from build123d import *

# Parameters (mm, degrees)
SKETCH2_R               = 1
CUT_EXTRUDE2_DEPTH      = 8.5
CUT_EXTRUDE2_DEPTH_BACK = 8.5


with BuildPart() as part:
    # Sketch1 → Revolve2 (revolve)
    with BuildSketch(Plane.XY):
        Polygon((-16.067192276, 0), (38.932807724, 0), (38.932807724, 2.992227979), (-12.067192276, 2.992227979), (-12.067192276, 7.5), (-16.067192276, 7.5), align=None)
    revolve(axis=Axis((-16.067192276, 0, 0), (1, 0, 0)))

    # Sketch2 → Cut-Extrude2 (cut, two sides)
    with BuildSketch(Plane.XY) as cut_extrude2_sk:
        with Locations((35.91188951, 0)):
            Circle(SKETCH2_R)
    extrude(amount=CUT_EXTRUDE2_DEPTH, mode=Mode.SUBTRACT)
    extrude(cut_extrude2_sk.sketch, amount=-CUT_EXTRUDE2_DEPTH_BACK, mode=Mode.SUBTRACT)


solid = part.part
Source: CAD feature listing. Evaluate the final solid. Frame: model axes, mm. A direction names the side the tool comes from. Round coordinates to 2 decimals unless told otherwise and drop trailing zeros. Order: outer loops, then holes, each group sorted by start corner. A loop starts at its lowest first (then second) coordinate and runs counter-clockwise, first axis right, second up. Notation, with made-up numbers: (59, -17.5) - (86, -17.5) arc R13 cw to (86, 1.5) - close; hole circle Ø5 at (63.25, 3). An arc over 180 degrees is marked (long way). Use a Markdown table: item, result. Add a question column.
1. Section query B-B (z = -2.5). Return the cut outline in (x, y).
2. Section query D-D (z = 2). Return the cut outline in (x, y).
3. Section query C-C (y = -4.5). Return the cut outline in (x, z), then the cut area to 3 significant figures.
4. Line query: probe 1 along X at (y, z) = (0, -0.75); probe 2 along X at (y, z) = (2.25, -5.25); probe 3 along Z at (x, y) = (-1, 0.25). Output: solid intervals per line, ascending.
5. Set-up query: faces 1 (the cylindrical face through (13.076, 2.854, 0.899)), 2 (the flat face through (-16.067, 0, 0)). Return all of +Z, -Z, +X, -X, +Y, -Y with unobstructed straight access to the full face (end or side cutting, diameter ignored); none if empty.
6. Section query A-A (y = 0). Return the cut outline in (x, z), then the cut area to 3 significant figures.
7. First-contact query: pin 1 (5 mm diameter, centred on x = -2, z = 0, fed in from +Y); pin 2 (4 mm diameter, centred on x = 13, z = -0.5, fed in from -Y); pin 3 (8 mm diameter, centred on y = -2.5, z = 5, fed in from +X); pin 4 (3 mm diameter, centred on x = 35.91, y = 0, fed in from -Z). Flat tips, straight axial feed; report the tip coordinate or a pass-through.
Derived:
| question | item | result |
|---|---|---|
| 1 | outline | (-16.07, -7.07) - (-12.07, -7.07) - (-12.07, -1.64) - (38.93, -1.64) - (38.93, 1.64) - (-12.07, 1.64) - (-12.07, 7.07) - (-16.07, 7.07) - close; hole circle Ø2 at (35.91, 0) |
| 2 | outline | (-16.07, -7.23) - (-12.07, -7.23) - (-12.07, -2.23) - (38.93, -2.23) - (38.93, 2.23) - (-12.07, 2.23) - (-12.07, 7.23) - (-16.07, 7.23) - close; hole circle Ø2 at (35.91, 0) |
| 3 | outline | (-16.07, -6) - (-12.07, -6) - (-12.07, 6) - (-16.07, 6) - close |
| 3 | area | 48.0 mm2 |
| 4 | probe 1 | -16.07 to 34.91, 36.91 to 38.93 |
| 4 | probe 2 | -16.07 to -12.07 |
| 4 | probe 3 | -2.98 to 2.98 |
| 5 | face 1 | +X |
| 5 | face 2 | +Z, -Z, -X, +Y, -Y |
| 6 | outline | (-16.07, -7.5) - (-12.07, -7.5) - (-12.07, -2.99) - (34.91, -2.99) - (34.91, 2.99) - (-12.07, 2.99) - (-12.07, 7.5) - (-16.07, 7.5) - close; (36.91, -2.99) - (38.93, -2.99) - (38.93, 2.99) - (36.91, 2.99) - close |
| 6 | area | 353 mm2 |
| 7 | pin 1 | y = 2.99 |
| 7 | pin 2 | y = -2.99 |
| 7 | pin 3 | x = 38.93 |
| 7 | pin 4 | z = -2.99 |
